from build123d import *

# Parameters (mm, degrees)
LOFT1_DEPTH        = 508
LOFT1_DRAFT        = -6.7116474
SHELL1_T           = -19.05
SKETCH5_R          = 147.867108762
CUT_EXTRUDE1_DEPTH = 17.78
CUT_EXTRUDE2_DEPTH = 528.39436013
CUT_EXTRUDE2_TAPER = -20


# Read off the part's stored shape, not the designer's step: Loft1
with BuildPart() as part:
    # Loft1 outline → Loft1 (with draft: the straight prism first)
    with BuildSketch(Plane(origin=(0, -508, 0), x_dir=(1, 0, 0), z_dir=(0, 1, 0))):
        Polygon((33.642737163, -58.270930071), (51.543663709, -43.250269208), (63.227663709, -23.012987572), (67.285474325, 0), (63.227663709, 23.012987572), (51.543663709, 43.250269208), (33.642737163, 58.270930071), (11.684, 66.26325678), (-11.684, 66.26325678), (-33.642737163, 58.270930071), (-51.543663709, 43.250269208), (-63.227663709, 23.012987572), (-67.285474325, 0), (-63.227663709, -23.012987572), (-51.543663709, -43.250269208), (-33.642737163, -58.270930071), (-11.684, -66.26325678), (11.684, -66.26325678), align=None)
    extrude(amount=LOFT1_DEPTH)
    # Loft1: the draft: its side faces are tilted about the plane it starts from
    loft1_sides = [part.faces().sort_by_distance(p)[0] for p in [
        (42.593200436, -254, 50.76059964),
        (57.385663709, -254, 33.13162839),
        (65.256569017, -254, 11.506493786),
        (65.256569017, -254, -11.506493786),
        (57.385663709, -254, -33.13162839),
        (42.593200436, -254, -50.76059964),
        (22.663368581, -254, -62.267093426),
        (0, -254, -66.26325678),
        (-22.663368582, -254, -62.267093426),
        (-42.593200436, -254, -50.76059964),
        (-57.385663709, -254, -33.13162839),
        (-65.256569017, -254, -11.506493786),
        (-65.256569017, -254, 11.506493786),
        (-57.385663709, -254, 33.13162839),
        (-42.593200436, -254, 50.76059964),
        (-22.663368581, -254, 62.267093426),
        (0, -254, 66.26325678),
        (22.663368582, -254, 62.267093426),
    ]]
    draft(loft1_sides, Plane(origin=(0, -508, 0), x_dir=(1, 0, 0), z_dir=(0, 1, 0)), LOFT1_DRAFT)

    # Shell1
    shell1_openings = [part.faces().sort_by_distance(p)[0] for p in [
        (0, 0, 0),
        (0, -508, 0),
    ]]
    offset(amount=SHELL1_T, openings=shell1_openings, kind=Kind.INTERSECTION)

    # Sketch5 → Cut-Extrude1 (cut)
    with BuildSketch(Plane.XZ.offset(508)):
        Circle(SKETCH5_R)
    extrude(amount=-CUT_EXTRUDE1_DEPTH, mode=Mode.SUBTRACT)

    # Sketch6 → Cut-Extrude2 (cut, through all)
    with BuildSketch(Plane(origin=(-55.116718082, -475.589831727, -9.718564486), x_dir=(0.17364817766692822, 0, -0.9848077530122085), z_dir=(-0.11509707458405294, -0.9931469114771136, -0.020294719649782803))):
        Polygon((-12.052935, 125.180446117), (-8.67072745, 106.130446117), (8.67072745, 106.130446117), (12.052935, 125.180446117), align=None)
    extrude(amount=CUT_EXTRUDE2_DEPTH, taper=CUT_EXTRUDE2_TAPER, mode=Mode.SUBTRACT)


solid = part.part
Model file for the job. Use its own axes, mm. A direction names the side the tool comes from. Give positions to 0.01 mm unless a question says otherwise; leave off trailing zeros. Order: outer loops, then holes, each group sorted by start corner. A loop starts at its lowest first (then second) coordinate and runs counter-clockwise, first axis right, second up. Notation, with made-up numbers: (80, 86.5) - (132, 86.5) arc R26 ccw to (132, 113.5) - close; hole circle Ø8 at (-25.75, -32.75). An arc over 180 degrees is marked (long way). Write item = value, one per line. Start each with the question number.
1. Two-plate mould, pull along X, no slides. Class faces 1 (the flat face through (-0.3, -248.5, 96.8)), 2 (the flat face through (-72.9, -194.07, 41.78)), 3 (the flat face through (-32.814, -248.542, -91.065)), 4 (the flat face through (61.98, -248.54, 74.35)): pulls with the +X half, pulls with the -X half, needs draft (parallel to the pull), parting line crosses it, or undercut.
2. Cut at B-B, the plane z = 88. List the corners of the cut face in (x, y).
3. Drop flat-ended pins along their axis: P1, Ø4, axis at y = -293, z = -42, coming from the -X side; P2, Ø5, axis at x = -83.5, y = -103, coming from the -Z side; P3, Ø8, axis at y = -101.5, z = -55.5, coming from the -X side. Give the stop position or say it passes through.
4. Probe line 1 along Z through (x, y) = (11.5, -207.5); line 2 along X through (y, z) = (-236, 61.5); line 3 along X through (y, z) = (-79, -19). List the from-to ranges inside material, lowest first.
5. Which spindle directions (+Z, -Z, +X, -X, +Y, -Y) get a long thin tool onto all of the face, cutting with end or side? Do faces 5 (the flat face through (54.21, -194.07, -64.2)), 6 (the flat face through (95.38, -248.54, -16.5)). Say none if no direction does.
6. Cut at A-A, the plane z = -12. List the corners of the cut face in (x, y).
Taken from the geometry:
q1.face_1 = needs draft
q1.face_2 = undercut
q1.face_3 = pulls with the -X half
q1.face_4 = pulls with the +X half
q2.outline = (-91.22, 0) - (-50.81, -220.72) - (-15.52, -323.29) - (15.52, -323.29) - (50.81, -220.72) - (91.22, 0) - (61.37, 0) - (50.81, -57.72) - (15.52, -160.29) - (-15.52, -160.29) - (-50.81, -57.72) - (-61.37, 0) - close
q3.P1 = -82.67
q3.P2 = -80.78
q3.P3 = -102.08
q4.line_1 = -101.63 to -82.44, 82.44 to 101.63
q4.line_2 = -77.97 to -49.75, 49.75 to 77.97
q4.line_3 = -115.2 to -95.72, 95.72 to 115.2
q5.face_5 = +Y
q5.face_6 = -Z, +X, -Y
q6.outline = (-125.87, 0) - (-67.29, -490.22) - (-47.82, -490.22) - (-106.4, 0) - close; (47.82, -490.22) - (67.29, -490.22) - (125.87, 0) - (106.4, 0) - close
